Input: part model. Units: mm. Frame: model coordinates. Face numbers are marked on the shaded views. A direction names the side the tool comes from. Give positions to 0.01 mm unless a question says otherwise; leave off trailing zeros. Loops run counter-clockwise (first coordinate to the right, second up) from the corner with the lowest first, then second, coordinate; pieces in that order, holes last. Notation, with made-up numbers: (88.5, 81) -> (100.5, 81) arc R12 cw to (100.5, 91) -> close; hole circle Ø10 at (-4.5, 47). An arc over 180 degrees is marked (long way). Answer in a Markdown table with one row per item. Add a question column.
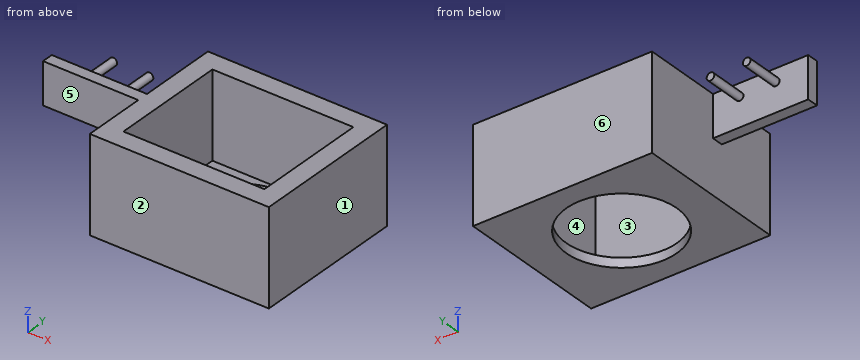
```python
from build123d import *

# Parameters (mm, degrees)
CROQUIS1_W                    = 47
CROQUIS1_H                    = 40.5
SALIENTE_EXTRUIR1_DEPTH       = 25
CROQUIS2_W                    = 10.933851529
CROQUIS2_H                    = 3
SALIENTE_EXTRUIR2_DEPTH       = 25
CROQUIS3_W                    = 37
CROQUIS3_H                    = 30.5
CORTAR_EXTRUIR1_DEPTH         = 22.5
CROQUIS4_W                    = 1
CROQUIS4_H                    = 10
CROQUIS5_W                    = 1
CROQUIS5_H                    = 10
TALADRO_DE_MARGEN_PARA_M251_D = 29


with BuildPart() as part:
    # Croquis1 → Saliente-Extruir1 (new body)
    with BuildSketch(Plane.XY.offset(25)):
        with Locations((-22.24307249, 34.18630066)):
            Rectangle(CROQUIS1_W, CROQUIS1_H)
    extrude(amount=-SALIENTE_EXTRUIR1_DEPTH)

    # Croquis2 → Saliente-Extruir2 (add)
    with BuildSketch(Plane.ZY.offset(45.74307249)):
        with Locations((19.533074236, 32.04630066)):
            Rectangle(CROQUIS2_W, CROQUIS2_H)
    extrude(amount=SALIENTE_EXTRUIR2_DEPTH)

    # Croquis3 → Cortar-Extruir1 (cut)
    with BuildSketch(Plane.XY.offset(25)):
        with Locations((-22.24307249, 34.18630066)):
            Rectangle(CROQUIS3_W, CROQUIS3_H)
    extrude(amount=-CORTAR_EXTRUIR1_DEPTH, mode=Mode.SUBTRACT)

    # Croquis4 → Revolución1 (revolve)
    with BuildSketch(Plane.XY.offset(21.590447053), mode=Mode.PRIVATE) as revoluci_n1_sk:
        with Locations((-52.24307249, 38.54630066)):
            Rectangle(CROQUIS4_W, CROQUIS4_H)
    revolve(revoluci_n1_sk.sketch.rotate(Axis((-52.74307249, 43.54630066, 21.590447053), (0, -1, 0)), 270), axis=Axis((-52.74307249, 43.54630066, 21.590447053), (0, -1, 0)))

    # Croquis5 → Revolución2 (revolve)
    with BuildSketch(Plane.XY.offset(21.590447053), mode=Mode.PRIVATE) as revoluci_n2_sk:
        with Locations((-61.74307249, 38.54630066)):
            Rectangle(CROQUIS5_W, CROQUIS5_H)
    revolve(revoluci_n2_sk.sketch.rotate(Axis((-62.24307249, 43.54630066, 21.590447053), (0, -1, 0)), 270), axis=Axis((-62.24307249, 43.54630066, 21.590447053), (0, -1, 0)))

    # Taladro de margen para M251 (through all)
    with Locations(Plane.XY.offset(2.5)):
        with Locations((-22.24307249, 34.18630066)):
            Hole(TALADRO_DE_MARGEN_PARA_M251_D / 2)


solid = part.part
```
1) Section D-D on y = 32.5. Output: boundary loops of the cut face in (x, z).
2) Pin query (flat end, axial travel): pin 1 (7 mm diameter, centred on y = 38, z = 17, fed in from -X); pin 2 (15 mm diameter, centred on x = -25, y = 31.5, fed in from +Z); pin 3 (5.5 mm diameter, centred on x = -53, z = 18, fed in from +Y); pin 4 (0.9 mm diameter, centred on x = -56.5, y = 32, fed in from -Z). Return the tip coordinate at first contact, or that it passes through.
3) Reachability of the marked faces 4, 5 and 6 from +Z, -Z, +X, -X, +Y, -Y: full face, straight path, thin tool, end or side. Return the list, or none.
4) Section C-C on x = -23.5. Output: boundary loops of the cut face in (y, z), and give its area (3 significant figures).
5) Material intervals for line 1 along Y through (x, z) = (-14.5, 13); line 2 along X through (y, z) = (23, 6.5); line 3 along X through (y, z) = (32.5, 17.25), sorted ascending.
6) Section B-B on z = 5.5. Output: boundary loops of the cut face in (x, y), and give its area (3 significant figures).
7) Pull-direction query (Y, two-part tool) for the marked faces 1, 2 and 3; classes: +Y half, -Y half, draft (parallel to the pull), parting line (faces both ways), or undercut.
8) Section A-A on y = 41. Output: boundary loops of the cut face in (x, z), and give its area (3 significant figures).
Working result:
| question | item | result |
|---|---|---|
| 1 | outline | (-70.74, 14.07) -> (-45.74, 14.07) -> (-45.74, 0) -> (-36.64, 0) -> (-36.64, 2.5) -> (-40.74, 2.5) -> (-40.74, 25) -> (-70.74, 25) -> close; (-7.84, 0) -> (1.26, 0) -> (1.26, 25) -> (-3.74, 25) -> (-3.74, 2.5) -> (-7.84, 2.5) -> close |
| 2 | pin 1 | stops at x = -45.74 |
| 2 | pin 2 | passes through |
| 2 | pin 3 | stops at y = 43.55 |
| 2 | pin 4 | stops at z = 14.07 |
| 3 | face 4 | +Z |
| 3 | face 5 | +Z, -Z, -X, -Y |
| 3 | face 6 | +Z, -Z, +X, -X, +Y |
| 4 | outline | (13.94, 0) -> (19.74, 0) -> (19.74, 2.5) -> (18.94, 2.5) -> (18.94, 25) -> (13.94, 25) -> close; (48.63, 0) -> (54.44, 0) -> (54.44, 25) -> (49.44, 25) -> (49.44, 2.5) -> (48.63, 2.5) -> close |
| 4 | area | 254 mm2 |
| 5 | line 1 | y = 13.94 to 18.94, 49.44 to 54.44 |
| 5 | line 2 | x = -45.74 to -40.74, -3.74 to 1.26 |
| 5 | line 3 | x = -70.74 to -40.74, -3.74 to 1.26 |
| 6 | outline | (-45.74, 13.94) -> (1.26, 13.94) -> (1.26, 54.44) -> (-45.74, 54.44) -> close; hole (-40.74, 18.94) -> (-3.74, 18.94) -> (-3.74, 49.44) -> (-40.74, 49.44) -> close |
| 6 | area | 775 mm2 |
| 7 | face 1 | draft |
| 7 | face 2 | -Y half |
| 7 | face 3 | undercut |
| 8 | outline | circle Ø2 at (-62.24, 21.59); circle Ø2 at (-52.74, 21.59); (-45.74, 0) -> (-35.04, 0) -> (-35.04, 2.5) -> (-40.74, 2.5) -> (-40.74, 25) -> (-45.74, 25) -> close; (-9.44, 0) -> (1.26, 0) -> (1.26, 25) -> (-3.74, 25) -> (-3.74, 2.5) -> (-9.44, 2.5) -> close |
| 8 | area | 285 mm2 |
